from build123d import *

# Parameters (mm, degrees)
BOSS_EXTRUDE1_DEPTH = 4.7625


with BuildPart() as part:
    # Sketch1 → Boss-Extrude1 (new body)
    with BuildSketch(Plane.XY.offset(4.7625)):
        with BuildLine():
            Line((-46.21916, -17.859375), (-14.676763422, -17.859375))
            ThreePointArc((-14.676763422, -17.859375), (-13.924040029, -17.612266731), (-13.464236596, -16.967103337))
            ThreePointArc((-13.464236596, -16.967103337), (-12.378086754, -15.44309532), (-10.6, -14.859375))
            Line((-10.6, -14.859375), (10.6, -14.859375))
            ThreePointArc((10.6, -14.859375), (12.378086754, -15.44309532), (13.464236596, -16.967103337))
            ThreePointArc((13.464236596, -16.967103337), (13.924040029, -17.612266731), (14.676763422, -17.859375))
            Line((14.676763422, -17.859375), (46.21916, -17.859375))
            ThreePointArc((46.21916, -17.859375), (47.117185612, -17.487400612), (47.48916, -16.589375))
            Line((47.48916, -16.589375), (47.48916, 16.589375))
            ThreePointArc((47.48916, 16.589375), (47.117185612, 17.487400612), (46.21916, 17.859375))
            Line((46.21916, 17.859375), (-46.21916, 17.859375))
            ThreePointArc((-46.21916, 17.859375), (-47.117185612, 17.487400612), (-47.48916, 16.589375))
            Line((-47.48916, 16.589375), (-47.48916, -16.589375))
            ThreePointArc((-47.48916, -16.589375), (-47.117185612, -17.487400612), (-46.21916, -17.859375))
        make_face()
        with BuildLine():
            Line((34.78916, -8.334375), (-34.78916, -8.334375))
            ThreePointArc((-34.78916, -8.334375), (-37.96416, -5.159375), (-34.78916, -1.984375))
            Line((-34.78916, -1.984375), (34.78916, -1.984375))
            ThreePointArc((34.78916, -1.984375), (37.96416, -5.159375), (34.78916, -8.334375))
        make_face(mode=Mode.SUBTRACT)
        with BuildLine():
            Line((34.8316655, 7.546875), (-34.7466545, 7.546875))
            ThreePointArc((-34.7466545, 7.546875), (-37.9216545, 10.721875), (-34.7466545, 13.896875))
            Line((-34.7466545, 13.896875), (34.8316655, 13.896875))
            ThreePointArc((34.8316655, 13.896875), (38.0066655, 10.721875), (34.8316655, 7.546875))
        make_face(mode=Mode.SUBTRACT)
    extrude(amount=-BOSS_EXTRUDE1_DEPTH)


solid = part.part
Could you check a few things on this model? Use its own coordinates, in mm. A direction names the side the tool comes from. Coordinates: 2 decimals unless noted, no trailing zeros. Loops run counter-clockwise (first coordinate to the right, second up) from the corner with the lowest first, then second, coordinate; pieces in that order, holes last.
1. Imagine slicing it at C-C (y = 9.5). Please give me the cut outline in (x, z), and give its area (3 significant figures).
2. Imagine slicing it at D-D (x = 33). Please give me the cut outline in (y, z).
3. I need wall thicknesses on L1, parallel to Y at x = -7, z = 0.85; L2, parallel to Y at x = -16.5, z = 3.05; L3, parallel to X at y = 10.5, z = 4.2. Which ranges of each line are inside material? Lowest first, please.
4. Imagine slicing it at B-B (x = 1). Please give me the cut outline in (y, z).
5. For faces 1 (the face through (-31, -17.859, 2)), 2 (the face through (0, -14.859, 2)), 3 (the face through (1, 7.547, 2)), which set-ups out of +Z, -Z, +X, -X, +Y, -Y let a thin tool reach every point of the face, with its end or its side?
6. We'd pull the mould along X, two halves only. Please class faces 4 (the face through (1, 17.859, 2)), 5 (the face through (47.489, 0, 2)), 6 (the face through (37.963, -5.09, 2.415)), 7 (the face through (-47.489, 0, 2)): released by +X, released by -X, zero draft, split by the parting line, or undercut.
7. For P1, Ø2.5, axis at x = 4, z = 3, coming from the -Y side, with a flat end and sliding along its axis, tell me the tip position at first contact or that it passes through.
8. Imagine slicing it at A-A (z = 3.7). Please give me the cut outline in (x, y) (3 decimals), and give its area (3 significant figures).
Computed values:
1. outline: (-47.49, 0) - (-37.68, 0) - (-37.68, 4.76) - (-47.49, 4.76) - close; (37.76, 0) - (47.49, 0) - (47.49, 4.76) - (37.76, 4.76) - close
1. area: 93.1 mm2
2. outline: (-17.86, 0) - (-8.33, 0) - (-8.33, 4.76) - (-17.86, 4.76) - close; (-1.98, 0) - (7.55, 0) - (7.55, 4.76) - (-1.98, 4.76) - close; (13.9, 0) - (17.86, 0) - (17.86, 4.76) - (13.9, 4.76) - close
3. L1: y = -14.86 to -8.33, -1.98 to 7.55, 13.9 to 17.86
3. L2: y = -17.86 to -8.33, -1.98 to 7.55, 13.9 to 17.86
3. L3: x = -47.49 to -37.91, 38 to 47.49
4. outline: (-14.86, 0) - (-8.33, 0) - (-8.33, 4.76) - (-14.86, 4.76) - close; (-1.98, 0) - (7.55, 0) - (7.55, 4.76) - (-1.98, 4.76) - close; (13.9, 0) - (17.86, 0) - (17.86, 4.76) - (13.9, 4.76) - close
5. face 1: +Z, -Z, +X, -X, -Y
5. face 2: +Z, -Z, -Y
5. face 3: +Z, -Z
6. face 4: zero draft
6. face 5: released by +X
6. face 6: undercut
6. face 7: released by -X
7. P1: stops at y = -14.86
8. outline: (-47.489, -16.589) arc R1.27 ccw to (-46.219, -17.859) - (-14.677, -17.859) arc R1.27 ccw to (-13.464, -16.967) arc R3 cw to (-10.6, -14.859) - (10.6, -14.859) arc R3 cw to (13.464, -16.967) arc R1.27 ccw to (14.677, -17.859) - (46.219, -17.859) arc R1.27 ccw to (47.489, -16.589) - (47.489, 16.589) arc R1.27 ccw to (46.219, 17.859) - (-46.219, 17.859) arc R1.27 ccw to (-47.489, 16.589) - close; hole (-34.789, -8.334) - (34.789, -8.334) arc R3.175 ccw to (34.789, -1.984) - (-34.789, -1.984) arc R3.175 ccw to start; hole (-34.747, 7.547) - (34.832, 7.547) arc R3.175 ccw to (34.832, 13.897) - (-34.747, 13.897) arc R3.175 ccw to start
8. area: 2,370 mm2
